Source: CAD feature listing. Evaluate the final solid. Frame: model axes, mm. A direction names the side the tool comes from. Round coordinates to 2 decimals unless told otherwise and drop trailing zeros. Order: outer loops, then holes, each group sorted by start corner. A loop starts at its lowest first (then second) coordinate and runs counter-clockwise, first axis right, second up. Notation, with made-up numbers: (69.5, -31.5) -> (91.5, -31.5) arc R14 ccw to (91.5, -21.5) -> close; hole circle Ø10 at (3.5, 38.25). An arc over 180 degrees is marked (long way). One line per item, written item: value. Start each with the question number.
1) Section A-A (x = 2.5). Return the cut outline in (y, z) (3 decimals), and give its area (3 significant figures).
2) Section B-B (y = 0.75). Return the cut outline in (x, z), and give its area (3 significant figures).
3) Mould query, pull axis Y, two halves, no side actions, for faces 1 (the face through (0, 2.667, 1)), 2 (the face through (0, 3.175, 1)), 3 (the face through (0, -2.667, 1)), 4 (the face through (0, 3, 0)). Classes: pulls with the +Y half, pulls with the -Y half, needs draft (parallel to the pull), parting line crosses it, or undercut.
4) Section D-D (z = 15.25). Return the cut outline in (x, y) (3 decimals).
5) Ray query, L1, parallel to Y at x = -6, z = 1.5 (3 decimals); L2, parallel to X at y = 1.75, z = 5.5; L3, parallel to X at y = -2.75, z = 14.5. Return the intervals inside material, ascending.
6) Pin query (flat end, axial travel): P1, Ø12, axis at x = 8.5, z = 12, coming from the +Y side (3 decimals); P2, Ø3, axis at x = -9.5, z = 18.5, coming from the -Y side; P3, Ø0.6, axis at x = 0.5, y = 3, coming from the +Z side; P4, Ø0.6, axis at x = 9, y = 3, coming from the +Z side. Return the tip coordinate at first contact, or that it passes through.
7) Section C-C (z = 3). Return the cut outline in (x, y) (3 decimals), and give its area (3 significant figures).
8) Reachability of faces 5 (the face through (-24.892, 0, 13)), 6 (the face through (-25.1, -0.2, 25.4)) from +Z, -Z, +X, -X, +Y, -Y: full face, straight path, thin tool, end or side. Return the list, or none.
```python
from build123d import *

# Parameters (mm, degrees)
F0_W     = 50.8
F0_H     = 6.35
F1_DEPTH = 25.4
F2_T     = -0.508
F3_W     = 6.35
F3_H     = 7.62
F3_W_2   = 12.7
F4_DEPTH = 13.208


with BuildPart() as f1:
    # F0 (on Top) → F1 (new body)
    with BuildSketch(Plane.XY):
        Rectangle(F0_W, F0_H)
    extrude(amount=F1_DEPTH)

    # F2
    f2_openings = [f1.faces().sort_by_distance(p)[0] for p in [
        (0, 0, 25.4),
        (0, 0, 0),
    ]]
    offset(amount=F2_T, openings=f2_openings)

    # F3 (on face) → F4 (cut)
    with BuildSketch(Plane.XZ.offset(3.175)):
        with Locations((-15.875, 21.59)):
            Rectangle(F3_W, F3_H)
        with Locations((-9.525, 21.59)):
            Rectangle(F3_W, F3_H)
        with Locations((0, 21.59)):
            Rectangle(F3_W_2, F3_H)
        with Locations((-9.525, 13.97)):
            Rectangle(F3_W, F3_H)
        with Locations((9.525, 21.59)):
            Rectangle(F3_W, F3_H)
        with Locations((0, 13.97)):
            Rectangle(F3_W_2, F3_H)
        with Locations((15.875, 21.59)):
            Rectangle(F3_W, F3_H)
        with Locations((9.525, 13.97)):
            Rectangle(F3_W, F3_H)
        with Locations((0, 6.35)):
            Rectangle(F3_W_2, F3_H)
    extrude(amount=-F4_DEPTH, mode=Mode.SUBTRACT)


solid = f1.part
```
Findings:
1. outline: (-3.175, 0) -> (-2.667, 0) -> (-2.667, 2.54) -> (-3.175, 2.54) -> close; (2.667, 0) -> (3.175, 0) -> (3.175, 2.54) -> (2.667, 2.54) -> close
1. area: 2.58 mm2
2. outline: (-25.4, 0) -> (-24.89, 0) -> (-24.89, 25.4) -> (-25.4, 25.4) -> close; (24.89, 0) -> (25.4, 0) -> (25.4, 25.4) -> (24.89, 25.4) -> close
2. area: 25.8 mm2
3. face 1: undercut
3. face 2: pulls with the +Y half
3. face 3: undercut
3. face 4: needs draft
4. outline: (-25.4, -3.175) -> (-12.7, -3.175) -> (-12.7, -2.667) -> (-24.892, -2.667) -> (-24.892, 2.667) -> (-12.7, 2.667) -> (-12.7, 3.175) -> (-25.4, 3.175) -> close; (12.7, -3.175) -> (25.4, -3.175) -> (25.4, 3.175) -> (12.7, 3.175) -> (12.7, 2.667) -> (24.892, 2.667) -> (24.892, -2.667) -> (12.7, -2.667) -> close
5. L1: -3.175 to -2.667, 2.667 to 3.175
5. L2: -25.4 to -24.89, 24.89 to 25.4
5. L3: -25.4 to -12.7, 12.7 to 25.4
6. P1: y = 3.175
6. P2: through
6. P3: z = 2.54
6. P4: z = 10.16
7. outline: (-25.4, -3.175) -> (-6.35, -3.175) -> (-6.35, -2.667) -> (-24.892, -2.667) -> (-24.892, 2.667) -> (-6.35, 2.667) -> (-6.35, 3.175) -> (-25.4, 3.175) -> close; (6.35, -3.175) -> (25.4, -3.175) -> (25.4, 3.175) -> (6.35, 3.175) -> (6.35, 2.667) -> (24.892, 2.667) -> (24.892, -2.667) -> (6.35, -2.667) -> close
7. area: 44.1 mm2
8. face 5: +Z, -Z
8. face 6: +Z, +X, -X, +Y, -Y
